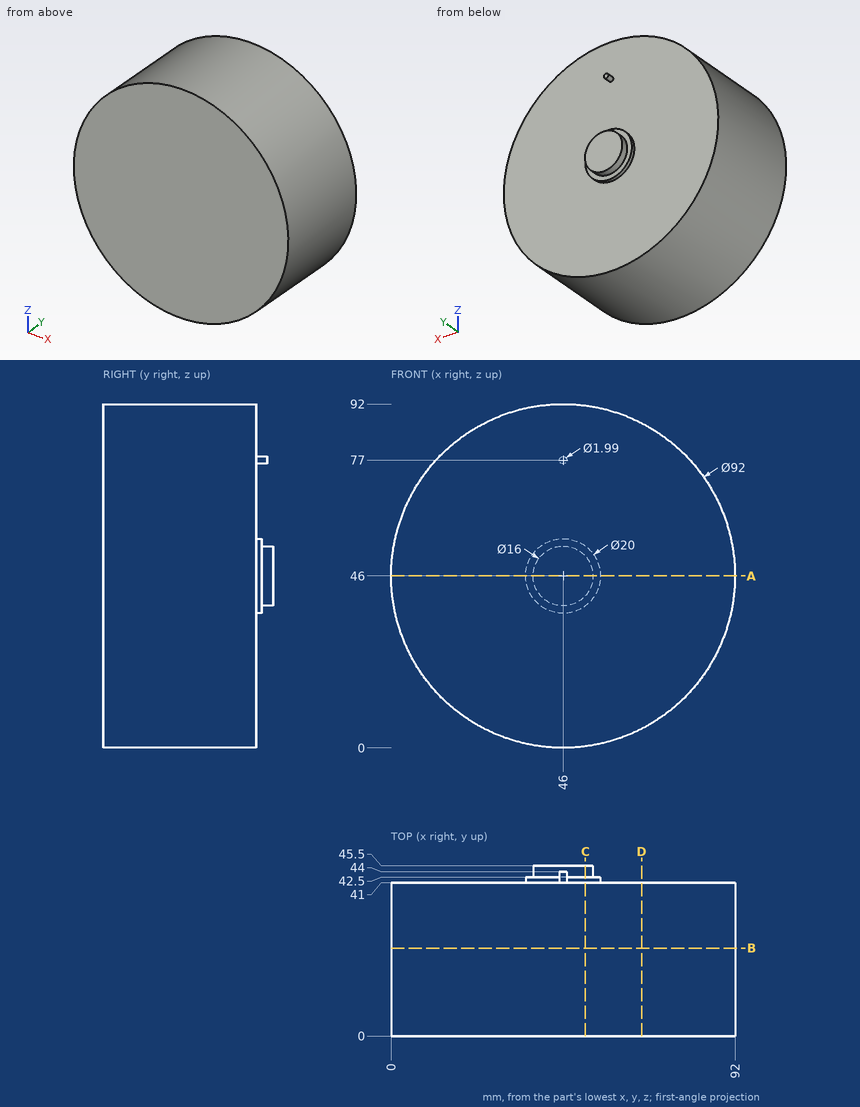
Source: three-view drawing plus pictorial views. Frame: mm from the lowest corner of the part. Coordinates: 2 decimals unless noted, no trailing zeros. Loops run counter-clockwise (first coordinate to the right, second up) from the corner with the lowest first, then second, coordinate; pieces in that order, holes last. Notation, with made-up numbers: (19.25, 31) -> (45.25, 31) arc R7 ccw to (45.25, 37) -> close; hole circle Ø7 at (56.5, 59.5). An arc over 180 degrees is marked (long way). Answer in a Markdown table with one row per item. Add a question column.
Q1. Ray query, line 1 along Y through (x, z) = (60.5, 33.5); line 2 along Z through (x, y) = (47.5, 28); line 3 along Y through (x, z) = (54, 42). Return the intervals inside material, ascending.
Q2. Contact query for flat-ended pins moving along their axis: pin 1 Ø1 at (y, z) = (35, 82.5) entering from +X; pin 2 Ø12 at (x, y) = (44, 12) entering from +Z; pin 3 Ø2 at (x, z) = (46.5, 74.5) entering from +Y; pin 4 Ø3 at (y, z) = (35, 61) entering from -X. Output: stop coordinate, or through.
Q3. Section D-D on x = 67. Return the cut outline in (y, z), and give its area (3 significant figures).
Q4. Section A-A on z = 46. Return the cut outline in (x, y), and give its area (3 significant figures).
Q5. Section B-B on y = 23.5. Return the cut outline in (x, z), and give its area (3 significant figures).
Q6. Section C-C on x = 52. Return the cut outline in (y, z), and give its area (3 significant figures).
Computed values:
| question | item | result |
|---|---|---|
| 1 | line 1 | y = 0 to 41 |
| 1 | line 2 | z = 0.02 to 91.98 |
| 1 | line 3 | y = 0 to 42.5 |
| 2 | pin 1 | stops at x = 74.64 |
| 2 | pin 2 | stops at z = 92 |
| 2 | pin 3 | stops at y = 41 |
| 2 | pin 4 | stops at x = 2.03 |
| 3 | outline | (0, 5.07) -> (41, 5.07) -> (41, 86.93) -> (0, 86.93) -> close |
| 3 | area | 3,360 mm^2 |
| 4 | outline | (0, 0) -> (92, 0) -> (92, 41) -> (56, 41) -> (56, 42.5) -> (54, 42.5) -> (54, 45.5) -> (38, 45.5) -> (38, 42.5) -> (36, 42.5) -> (36, 41) -> (0, 41) -> close |
| 4 | area | 3,850 mm^2 |
| 5 | outline | circle Ø92 at (46, 46) |
| 5 | area | 6,650 mm^2 |
| 6 | outline | (0, 0.39) -> (41, 0.39) -> (41, 38) -> (42.5, 38) -> (42.5, 40.71) -> (45.5, 40.71) -> (45.5, 51.29) -> (42.5, 51.29) -> (42.5, 54) -> (41, 54) -> (41, 91.61) -> (0, 91.61) -> close |
| 6 | area | 3,800 mm^2 |
